from build123d import *

# Parameters (mm, degrees)
SKETCH1_W                                     = 220
SKETCH1_H                                     = 12
SKETCH1_R                                     = 1.7
SKETCH1_R_2                                   = 3.3
HEADER_CROSSBEAM_DEPTH                        = 6
SKETCH2_R                                     = 1.7
BENCH_HEADER_M3_CLEARANCE_HOLES_2X_D3P4_DEPTH = 6.5


with BuildPart() as part:
    # Sketch1 → Header_Crossbeam (new body)
    with BuildSketch(Plane.XY):
        Rectangle(SKETCH1_W, SKETCH1_H)
        with Locations((-105, 0)):
            Circle(SKETCH1_R, mode=Mode.SUBTRACT)
        with Locations((105, 0)):
            Circle(SKETCH1_R, mode=Mode.SUBTRACT)
        with Locations((-42, 0)):
            Circle(SKETCH1_R_2, mode=Mode.SUBTRACT)
        with Locations((42, 0)):
            Circle(SKETCH1_R_2, mode=Mode.SUBTRACT)
    extrude(amount=HEADER_CROSSBEAM_DEPTH)

    # Sketch2 → Bench_Header_M3_Clearance_Holes_2x_D3p4 (cut)
    with BuildSketch(Plane.XY.offset(6)):
        with Locations((-20, 0)):
            Circle(SKETCH2_R)
        with Locations((20, 0)):
            Circle(SKETCH2_R)
    extrude(amount=-BENCH_HEADER_M3_CLEARANCE_HOLES_2X_D3P4_DEPTH, mode=Mode.SUBTRACT)


solid = part.part
Can you work these out from the model? Positions are in its coordinate system, mm. Give positions to 0.01 mm unless a question says otherwise; leave off trailing zeros. Loops run counter-clockwise (first coordinate to the right, second up) from the corner with the lowest first, then second, coordinate; pieces in that order, holes last. Notation, with made-up numbers: (57, 80) - (67, 80) arc R15 cw to (67, 108) - close; hole circle Ø1 at (-2.5, 7). An arc over 180 degrees is marked (long way). Return JSON: item names as keys, results as strings.
1. I'm going to push a flat-ended pin straight in: pin 1 Ø6 at (x, y) = (42, 0) entering from -Z. Where does the tip first touch, or does it pass through?
Output values:
{"pin 1": "passes through"}
2. We'd pull the mould along Y, two halves only. Please class faces 1 (the face through (21.57, -0.65, 3.04)), 2 (the face through (-2, 6, 3)), 3 (the face through (-110, 0, 3)): +Y half, -Y half, draft (parallel to the pull), parting line (faces both ways), or undercut.
Output values:
{"face 1": "undercut", "face 2": "+Y half", "face 3": "draft"}
3. I want a section at B-B on z = 3.6. Please give me the cut outline in (x, y), and give its area (3 significant figures).
Output values:
{"outline": "(-110, -6) - (110, -6) - (110, 6) - (-110, 6) - close; hole circle Ø3.4 at (-105, 0); hole circle Ø6.6 at (-42, 0); hole circle Ø3.4 at (-20, 0); hole circle Ø3.4 at (20, 0); hole circle Ø6.6 at (42, 0); hole circle Ø3.4 at (105, 0)", "area": "2,540 mm²"}
4. I want a section at A-A on x = 42. Please give me the cut outline in (y, z), and give its area (3 significant figures).
Output values:
{"outline": "(-6, 0) - (-3.3, 0) - (-3.3, 6) - (-6, 6) - close; (3.3, 0) - (6, 0) - (6, 6) - (3.3, 6) - close", "area": "32.4 mm²"}
5. If I drill on line 1 (Y direction, x = -42, z = 2.05); line 2 (Y direction, x = -105, z = 3.6); line 3 (X direction, y = -2.25, z = 2.15), over which ranges is the centre line in solid material (lowest first)?
Output values:
{"line 1": "y = -6 to -3.3, 3.3 to 6", "line 2": "y = -6 to -1.7, 1.7 to 6", "line 3": "x = -110 to -44.41, -39.59 to 39.59, 44.41 to 110"}
